Check sheet for the modelled part. Datum: model origin and axes. Units: mm. A direction names the side the tool comes from. Round coordinates to 2 decimals unless told otherwise and drop trailing zeros. Order: outer loops, then holes, each group sorted by start corner. A loop starts at its lowest first (then second) coordinate and runs counter-clockwise, first axis right, second up.
Q1. Mould release check, pull along Y, two halves, no side actions. Record for faces 1 (the cylindrical face through (4.831, 12.082, 22.133)), 2 (the flat face through (7, -10.5, 0)), 3 (the flat face through (9.8, -11, 7)): +Y half, -Y half, draft (parallel to the pull), parting line (faces both ways), or undercut.
Q2. Cross-section at C-C on x = 3. Record the cut outline in (y, z).
Q3. Cross-section at A-A on x = 9. Record the cut outline in (y, z).
Q4. Set-up check for faces 4 (the flat face through (5, 11.5, 26)), 5 (the flat face through (7, 10.5, 0)), 6 (the flat face through (5, 0, 23.7)), 7 (the flat face through (5, -5, 26)), 8 (the flat face through (5, -13, 16.2)): record each of +Z, -Z, +X, -X, +Y, -Y from which the full face is reachable in a straight line by a thin tool's end or side.
Q5. Cross-section at B-B on z = -19.2. Record the cut outline in (x, y).
Q6. Cross-section at D-D on y = 9.5. Record the cut outline in (x, z), then the cut area to 3 significant figures.
Q7. Scan lines: probe 1 along Y at (x, z) = (4, 24); probe 2 along Y at (x, z) = (6, -5.5); probe 3 along Y at (x, z) = (8.5, 18). Record each from-to range of solid material in increasing order.
Q8. Depth check by flat-ended pin: P1, Ø5, axis at x = 7, z = -13, coming from the -Y side; P2, Ø1, axis at x = 5, z = 26, coming from the +Y side; P3, Ø6.5, axis at y = -3.5, z = -4, coming from the +X side. Enter the tip coordinate at first touch or a pass-through.
from build123d import *

# Parameters (mm, degrees)
SKETCH024_W     = 27
SKETCH024_H     = 55.4
PAD006_DEPTH    = 9.8
SKETCH025_W     = 21
SKETCH025_H     = 55.4
POCKET022_DEPTH = 6
SKETCH026_W     = 10
SKETCH026_H     = 4
PAD007_DEPTH    = 2
SKETCH027_R     = 2
PAD008_DEPTH    = 6
SKETCH028_W     = 2
SKETCH028_H     = 43.9
POCKET023_DEPTH = 9.8
SKETCH029_W     = 48.033568
SKETCH029_H     = 4.9
PAD009_DEPTH    = 3.4


with BuildPart() as part:
    # Sketch024 → Pad006 (new body)
    with BuildSketch(Plane.YZ):
        Rectangle(SKETCH024_W, SKETCH024_H)
    extrude(amount=PAD006_DEPTH)

    # Sketch025 (on Face6 of Pad006) → Pocket022 (cut)
    with BuildSketch(Plane.YZ.offset(9.8)):
        Rectangle(SKETCH025_W, SKETCH025_H)
    extrude(amount=-POCKET022_DEPTH, mode=Mode.SUBTRACT)

    # Sketch026 (on Face6 of Pocket022) → Pad007 (join)
    with BuildSketch(Plane.YZ.offset(3.8)):
        with Locations((0, 25.7)):
            Rectangle(SKETCH026_W, SKETCH026_H)
    extrude(amount=PAD007_DEPTH)

    # Sketch027 (on Face6 of Pad007) → Pad008 (join)
    with BuildSketch(Plane.YZ.offset(3.8)):
        with Locations((-5, -19.2)):
            Circle(SKETCH027_R)
    extrude(amount=PAD008_DEPTH)

    # Sketch028 (on Face2 of Pad008) → Pocket023 (cut)
    with BuildSketch(Plane(origin=(0, 0, 0), x_dir=(0, 1, 0), z_dir=(-1, 0, 0))):
        with Locations((-12.5, 5.75)):
            Rectangle(SKETCH028_W, SKETCH028_H)
        with BuildLine():
            ThreePointArc((13.5, -21.333568), (12.06697, -22.150807), (11.5, -23.7))
            Line((11.5, -23.7), (11.5, -27.7))
            Line((11.5, -27.7), (13.5, -27.7))
            Line((13.5, -27.7), (13.5, -21.333568))
        make_face()
    extrude(amount=-POCKET023_DEPTH, mode=Mode.SUBTRACT)

    # Sketch029 (on Face3 of Pocket023) → Pad009 (join)
    with BuildSketch(Plane.ZX.offset(13.5)):
        with Locations((-3.683216, 2.45)):
            Rectangle(SKETCH029_W, SKETCH029_H)
    extrude(amount=PAD009_DEPTH)


solid = part.part
Results found:
1. face 1: +Y half
1. face 2: undercut
1. face 3: draft
2. outline: (-13.5, 16.2) - (-11.5, 16.2) - (-11.5, -27.7) - (16.9, -27.7) - (16.9, 20.33) - (13.5, 20.33) - (13.5, 21.33) arc R2.4 cw to (11.5, 23.7) - (11.5, 27.7) - (-13.5, 27.7) - close
3. outline: (-13.5, 16.2) - (-11.5, 16.2) - (-11.5, -27.7) - (-10.5, -27.7) - (-10.5, 27.7) - (-13.5, 27.7) - close; circle Ø4 at (-5, -19.2); (10.5, -27.7) - (13.5, -27.7) - (13.5, 21.33) arc R2.4 cw to (11.5, 23.7) - (11.5, 27.7) - (10.5, 27.7) - close
4. face 4: +Z, +X, -X, +Y
4. face 5: +Z, -Z, +X
4. face 6: +X
4. face 7: +Z, +X
4. face 8: -Z, +X, -X, -Y
5. outline: (0, -11.5) - (9.8, -11.5) - (9.8, -10.5) - (3.8, -10.5) - (3.8, -7) - (9.8, -7) - (9.8, -3) - (3.8, -3) - (3.8, 10.5) - (9.8, 10.5) - (9.8, 13.5) - (4.9, 13.5) - (4.9, 16.9) - (0, 16.9) - close
6. outline: (0, -27.7) - (3.8, -27.7) - (3.8, 27.7) - (0, 27.7) - close
6. area: 211 mm2
7. probe 1: y = -13.5 to -10.5, -5 to 5, 10.5 to 11.5
7. probe 2: y = -11.5 to -10.5, 10.5 to 13.5
7. probe 3: y = -13.5 to -10.5, 10.5 to 13.5
8. P1: stops at y = -11.5
8. P2: stops at y = 11.5
8. P3: stops at x = 3.8
